Job drawing, mm, ordinate dimensions from the low corner. One solid piece. Coordinates: 2 decimals unless noted, no trailing zeros. Loops run counter-clockwise (first coordinate to the right, second up) from the corner with the lowest first, then second, coordinate; pieces in that order, holes last. Notation, with made-up numbers: (-7, 50.5) - (4, 50.5) arc R36 ccw to (4, 85.5) - close; hole circle Ø9 at (80.25, 64). An arc over 180 degrees is marked (long way). One line per question, with ' | ' between items. Start each with the question number.
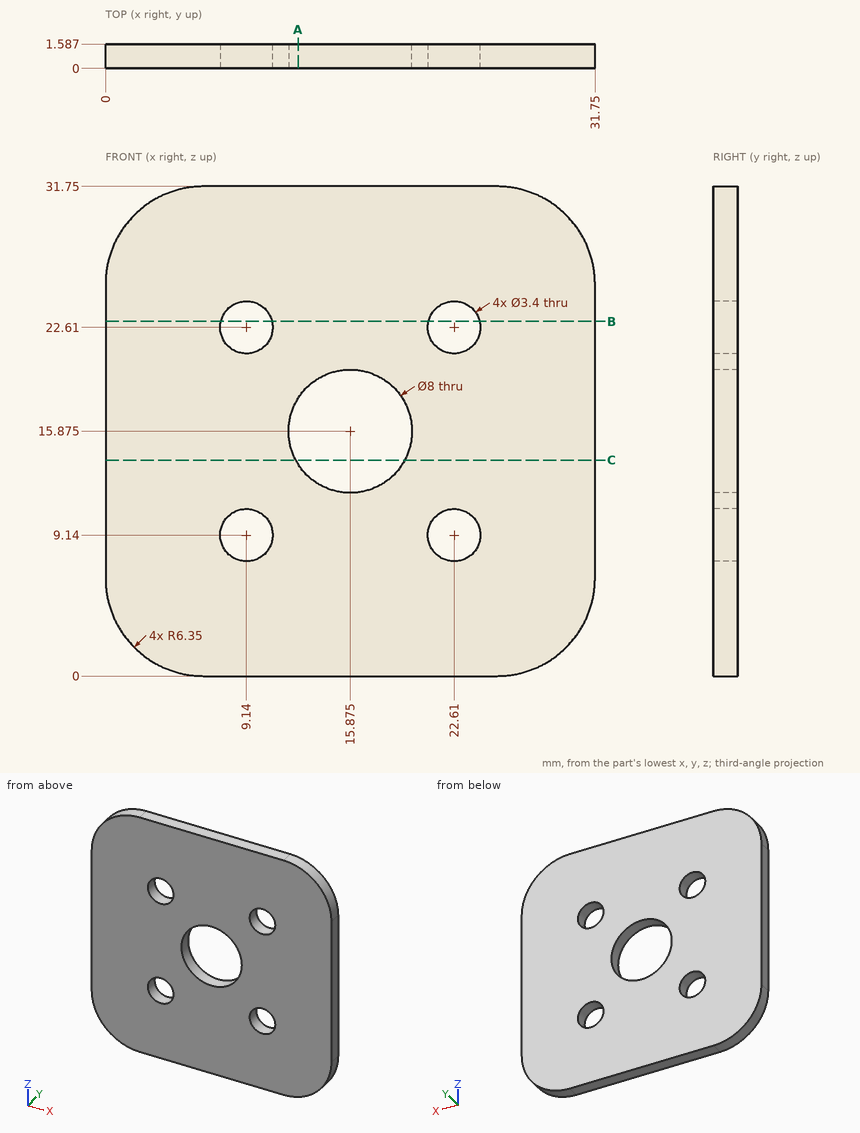
1) Band-saw the part on C-C on z = 14. List the corners of the cut face in (x, y).
2) Band-saw the part on A-A on x = 12.5. List the corners of the cut face in (y, z).
3) Band-saw the part on B-B on z = 23. Count the separate pieces of the cut face and the enclosed holes in it.
4) Wall check: line 1 along X through (y, z) = (0.2, 8); line 2 along Z through (x, y) = (15.5, 0.95); line 3 along X through (y, z) = (0.55, 4). Give the ranges that are in metal, low to high. Write a range as [from, to].
5) Pin check, flat tip, straight feed: pin 1 Ø2.5 at (x, z) = (9.14, 9.14) entering from +Y. Stop position of the tip, or through.
Values found:
1) outline: (0, 0) - (12.34, 0) - (12.34, 1.59) - (0, 1.59) - close; (19.41, 0) - (31.75, 0) - (31.75, 1.59) - (19.41, 1.59) - close
2) outline: (0, 0) - (1.59, 0) - (1.59, 13.73) - (0, 13.73) - close; (0, 18.02) - (1.59, 18.02) - (1.59, 31.75) - (0, 31.75) - close
3) separate pieces: 3 | enclosed holes: 0
4) line 1: [0, 7.88], [10.4, 21.35], [23.87, 31.75] | line 2: [0, 11.89], [19.86, 31.75] | line 3: [0.45, 31.3]
5) pin 1: through
